from build123d import *

# Parameters (mm, degrees)
BASE_FLANGE1_DEPTH     = 14
M3_CLEARANCE_HOLE1_D   = 3.4
M2_5_CLEARANCE_HOLE1_D = 2.9
SKETCH10_R             = 11.05
CUT_EXTRUDE1_DEPTH     = 10
SKETCH11_R             = 3
BOSS_EXTRUDE1_DEPTH    = 1.5
M3_CLEARANCE_HOLE2_D   = 3.4
SKETCH14_W             = 9
SKETCH14_H             = 16
SKETCH14_R             = 1.5
BOSS_EXTRUDE2_DEPTH    = 1.5
SKETCH15_W             = 28
SKETCH15_H             = 4
BOSS_EXTRUDE3_DEPTH    = 1.5
FILLET1_R              = 2
CUT_EXTRUDE2_DEPTH     = 10


# Sheet-metal steps are written as plain solids
with BuildPart() as part:
    # Sketch1 → Base-Flange1 (new, symmetric)
    with BuildSketch(Plane.XY):
        with BuildLine():
            Line((0, -24), (0, -1.5))
            ThreePointArc((0, -1.5), (0.439339828, -0.439339828), (1.5, 0))
            Line((1.5, 0), (32, 0))
            Line((32, 0), (32, 1.5))
            Line((32, 1.5), (1.5, 1.5))
            ThreePointArc((1.5, 1.5), (-0.621320344, 0.621320344), (-1.5, -1.5))
            Line((-1.5, -1.5), (-1.5, -24))
            Line((-1.5, -24), (0, -24))
        make_face()
    extrude(amount=BASE_FLANGE1_DEPTH, both=True)

    # M3 Clearance Hole1 (through all)
    with Locations(Plane.ZY.offset(1.5)):
        with Locations((-5, -5.25), (-5, -20.25), (5, -5.25), (5, -20.25)):
            Hole(M3_CLEARANCE_HOLE1_D / 2)

    # M2.5 Clearance Hole1 (through all)
    with Locations(Plane(origin=(0, 1.5, 0), x_dir=(1, 0, 0), z_dir=(0, 1, 0))):
        with Locations((29, 11.5), (29, -11.5), (6, -11.5), (6, 11.5)):
            Hole(M2_5_CLEARANCE_HOLE1_D / 2)

    # Sketch10 → Cut-Extrude1 (cut)
    with BuildSketch(Plane(origin=(0, 1.5, 0), x_dir=(1, 0, 0), z_dir=(0, 1, 0))):
        with Locations(Location((17.5, 0, 0), (0, 0, 270))):
            Circle(SKETCH10_R)
    extrude(amount=-CUT_EXTRUDE1_DEPTH, mode=Mode.SUBTRACT)

    # Sketch11 → Boss-Extrude1 (add)
    with BuildSketch(Plane(origin=(0, 1.5, 0), x_dir=(1, 0, 0), z_dir=(0, 1, 0))):
        Polygon((32, -14), (1.5, -14), (1.5, -24.597), (17.5, -24.597), (32, -24.597), align=None)
        with Locations(Location((17.5, -19.597, 0), (0, 0, 270))):
            Circle(SKETCH11_R, mode=Mode.SUBTRACT)
    extrude(amount=-BOSS_EXTRUDE1_DEPTH)

    # M3 Clearance Hole2 (through all)
    with Locations(Plane(origin=(0, 0, 0), x_dir=(-1, 0, 0), z_dir=(0, -1, 0))):
        with Locations((-26.5, -19.597), (-8.5, -19.597)):
            Hole(M3_CLEARANCE_HOLE2_D / 2)

    # Sketch14 → Boss-Extrude2 (add)
    with BuildSketch(Plane(origin=(0, 0, 0), x_dir=(0, 0, -1), z_dir=(1, 0, 0))):
        with Locations((18.5, -12.75)):
            Rectangle(SKETCH14_W, SKETCH14_H)
        with Locations((20, -7.75)):
            Circle(SKETCH14_R, mode=Mode.SUBTRACT)
        with Locations((20, -17.75)):
            Circle(SKETCH14_R, mode=Mode.SUBTRACT)
    boss_extrude2 = extrude(amount=-BOSS_EXTRUDE2_DEPTH)

    # Mirror1: Boss-Extrude2 across plane
    add(boss_extrude2.mirror(Plane.XY))

    # Sketch15 → Boss-Extrude3 (add)
    with BuildSketch(Plane(origin=(0, 0, 0), x_dir=(0, 0, -1), z_dir=(1, 0, 0))):
        with Locations((0, -26)):
            Rectangle(SKETCH15_W, SKETCH15_H)
    extrude(amount=-BOSS_EXTRUDE3_DEPTH)

    # Fillet1
    fillet1_edges = [part.edges().sort_by_distance(p)[0] for p in [
        (-0.75, -20.75, -14),
        (-0.75, -4.75, -14),
        (-0.75, -4.75, -23),
        (-0.75, -20.75, -23),
        (-0.75, -4.75, 14),
        (-0.75, -20.75, 14),
        (-0.75, -20.75, 23),
        (-0.75, -4.75, 23),
        (-0.75, -28, 14),
        (-0.75, -28, -14),
        (1.5, 0.75, 24.597),
        (32, 0.75, 24.597),
        (32, 0.75, -14),
    ]]
    fillet(fillet1_edges, radius=FILLET1_R)

    # Sketch16 → Cut-Extrude2 (cut)
    with BuildSketch(Plane(origin=(0, 0, 0), x_dir=(0, 0, -1), z_dir=(1, 0, 0))):
        with BuildLine():
            Line((-9, -10.25), (9, -10.25))
            ThreePointArc((9, -10.25), (11.5, -12.75), (9, -15.25))
            Line((9, -15.25), (-9, -15.25))
            ThreePointArc((-9, -15.25), (-11.5, -12.75), (-9, -10.25))
        make_face()
    extrude(amount=-CUT_EXTRUDE2_DEPTH, mode=Mode.SUBTRACT)


solid = part.part
Read the model definition and answer for the solid it produces. Units are mm, in the model's axes. A direction names the side the tool comes from. Round coordinates to 2 decimals unless told otherwise and drop trailing zeros. Loops run counter-clockwise (first coordinate to the right, second up) from the corner with the lowest first, then second, coordinate; pieces in that order, holes last. Notation, with made-up numbers: (14, 2) - (54, 2) arc R20 cw to (54, 11) - close; hole circle Ø3 at (-25, 38.25). An arc over 180 degrees is marked (long way). One line per question, with ' | ' between items. Start each with the question number.
Q1. Section B-B on z = -20 is taken. Give the vertices of the cut face in (x, y), plus the area to 3 significant figures.
Q2. Section A-A on y = -12.75 is taken. Give the vertices of the cut face in (x, z).
Q3. For faces 1 (the flat face through (-1, -20.75, 18)), 2 (the cylindrical face through (-0.74, -8.66, 18.81)), 3 (the flat face through (1.5, 1, 18)), 4 (the flat face through (10, 0, 9)), determine the directions among +Z, -Z, +X, -X, +Y, -Y from which every point of the face is accessible in a straight line to the end or side of a thin tool.
Q4. For a pull along Y with two mould halves and no side action, classify faces 5 (the cylindrical face through (-0.74, -8.66, -18.81)), 6 (the cylindrical face through (27.41, 0.76, 18.16)), 7 (the cylindrical face through (-0.7, -12.7, -11.5)), 8 (the cylindrical face through (-0.6, 0.64, 0.2)) as +Y half, -Y half, draft (parallel to the pull), parting line (faces both ways), or undercut.
Q5. Section D-D on z = 5 is taken. Give the vertices of the cut face in (x, y).
Q6. Flat-ended cylindrical pins translate along their axes: pin 1 (5 mm diameter, centred on x = 28, z = -11, fed in from -Y); pin 2 (0.8 mm diameter, centred on x = -0.5, y = -24.5, fed in from +Z); pin 3 (4.5 mm diameter, centred on y = -5.25, z = 5, fed in from +X). Find the tip coordinate at first contact, or state that the pin passes through.
Q7. Section C-C on y = -7.75 is taken. Give the vertices of the cut face in (x, z).
Q8. Find the intervals of material crossed by L1, parallel to Y at x = -1.1, z = 20; L2, parallel to X at y = 0.5, z = 11.5; L3, parallel to X at y = -5, z = 16, in increasing order.
Established:
1) outline: (-1.5, -20.75) - (0, -20.75) - (0, -19.25) - (-1.5, -19.25) - close; (-1.5, -16.25) - (0, -16.25) - (0, -9.25) - (-1.5, -9.25) - close; (-1.5, -6.25) - (0, -6.25) - (0, -4.75) - (-1.5, -4.75) - close | area: 15.0 mm²
2) outline: (-1.5, -23) - (0, -23) - (0, -11.5) - (-1.5, -11.5) - close; (-1.5, 11.5) - (0, 11.5) - (0, 23) - (-1.5, 23) - close
3) face 1: +Z, +X, -X, -Y | face 2: +X, -X | face 3: +Z, -X, +Y, -Y | face 4: +Z, -Z, +X, -Y
4) face 5: undercut | face 6: draft | face 7: undercut | face 8: +Y half
5) outline: (-1.5, -28) - (0, -28) - (0, -21.95) - (-1.5, -21.95) - close; (-1.5, -18.55) - (0, -18.55) - (0, -15.25) - (-1.5, -15.25) - close; (-1.5, -10.25) - (0, -10.25) - (0, -6.95) - (-1.5, -6.95) - close; (-1.5, -3.55) - (0, -3.55) - (0, -1.5) arc R1.5 cw to (1.5, 0) - (7.65, 0) - (7.65, 1.5) - (1.5, 1.5) arc R3 ccw to (-1.5, -1.5) - close; (27.35, 0) - (32, 0) - (32, 1.5) - (27.35, 1.5) - close
6) pin 1: y = 0 | pin 2: z = 14 | pin 3: x = 0
7) outline: (-1.5, -23) - (0, -23) - (0, -21.5) - (-1.5, -21.5) - close; (-1.5, -18.5) - (0, -18.5) - (0, 18.5) - (-1.5, 18.5) - close; (-1.5, 21.5) - (0, 21.5) - (0, 23) - (-1.5, 23) - close
8) L1: -20.75 to -19.25, -16.25 to -9.25, -6.25 to -4.75 | L2: -0.74 to 4.55, 7.45 to 27.55, 30.45 to 32 | L3: -1.5 to 0
